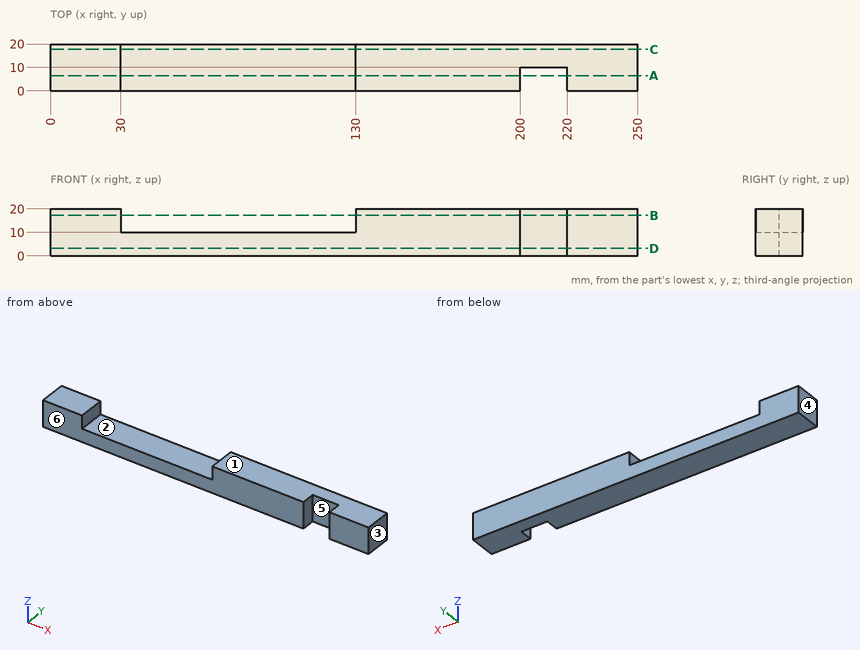
Part print with two shaded views. Sizes in mm from the minimum x, y, z corner. A direction names the side the tool comes from. Round coordinates to 2 decimals unless told otherwise and drop trailing zeros. Write each loop counter-clockwise with the first axis right and the second up, starting at its lowest first coordinate (ties: lowest second). Pieces come first, ordered by that corner, then holes. Notation, with made-up numbers: M 36,69.5 L 88,69.5 A10 cw 88,80.5 Z; hole C 26,19.25 d4. An arc over 180 degrees is marked long. Put each result on its own line as item: value. Start each with the question number.
1) 3-axis set-ups, long thin cutter, end or side, ignore diameter. For the marked faces 1 and 2: which of +Z, -Z, +X, -X, +Y, -Y reach the whole face in a straight line?
2) Saw through at C-C, the plane y = 17.75. Write the cut outline in (x, z).
3) Saw through at B-B, the plane z = 17.25. Write the cut outline in (x, y), and give its area (3 significant figures).
4) Drill centre lines: probe 1 along X at (y, z) = (2, 17.75); probe 2 along X at (y, z) = (7.5, 2.75); probe 3 along X at (y, z) = (18.5, 14.5). Where is each one in solid material? Low to high. Write a range as [from, to].
5) Pull direction X, two halves, no side cores. Call the marked faces 3, 4, 5 and 6: pulls with the +X half, pulls with the -X half, needs draft (parallel to the pull), parting line crosses it, or undercut.
6) Pin check, flat tips, straight feed: pin 1 Ø10 at (x, z) = (206, 6) entering from -Y; pin 2 Ø5 at (x, y) = (99, 3.5) entering from +Z. Stop position of each tip, or through.
7) Saw through at D-D, the plane z = 3.25. Write the cut outline in (x, y).
8) Saw through at A-A, the plane y = 6.5. Write the cut outline in (x, z), and give its area (3 significant figures).
Resolved:
1. face 1: +Z, +X, -X, +Y, -Y
1. face 2: +Z, +Y, -Y
2. outline: M 0,0 L 250,0 L 250,20 L 130,20 L 130,10 L 30,10 L 30,20 L 0,20 Z
3. outline: M 0,0 L 30,0 L 30,20 L 0,20 Z; M 130,0 L 200,0 L 200,10 L 220,10 L 220,0 L 250,0 L 250,20 L 130,20 Z
3. area: 2,800 mm²
4. probe 1: [0, 30], [130, 200], [220, 250]
4. probe 2: [0, 200], [220, 250]
4. probe 3: [0, 30], [130, 250]
5. face 3: pulls with the +X half
5. face 4: pulls with the -X half
5. face 5: undercut
5. face 6: needs draft
6. pin 1: y = 10
6. pin 2: z = 10
7. outline: M 0,0 L 200,0 L 200,10 L 220,10 L 220,0 L 250,0 L 250,20 L 0,20 Z
8. outline: M 0,0 L 200,0 L 200,20 L 130,20 L 130,10 L 30,10 L 30,20 L 0,20 Z; M 220,0 L 250,0 L 250,20 L 220,20 Z
8. area: 3,600 mm²
